Build history of the part. All positions in model axes, mm. A direction names the side the tool comes from. Round coordinates to 2 decimals unless told otherwise and drop trailing zeros. Loops run counter-clockwise (first coordinate to the right, second up) from the corner with the lowest first, then second, coordinate; pieces in that order, holes last. Notation, with made-up numbers: (-29, -5.5) - (-13, -5.5) arc R25 ccw to (-13, 27.5) - close; hole circle Ø8 at (-27, 45). An arc over 180 degrees is marked (long way). One line per question, with ' | ' between items. Start each with the question number.
Autodesk Inventor part; units mm, degrees
ref_plane "YZ Plane" through (0, 0, 0) normal (1, 0, 0) x (0, 1, 0)
ref_plane "XZ Plane" through (0, 0, 0) normal (0, 1, 0) x (-1, 0, 0)
ref_plane "XY Plane" through (0, 0, 0) normal (0, 0, 1) x (1, 0, 0)
sketch "Sketch1" plane through (0, 0, 0) normal (0, 0, 1) x (1, 0, 0)
  circle A0 centre (0, 0) radius 6
  dimension "d0" = 12
extrude "Extrusion1" add sketch "Sketch1" along normal blind 35
sketch "Sketch2" plane through (0, 0, 35) normal (0, 0, 1) x (1, 0, 0)
  circle A0 centre (0, 0) radius 2
  circle A1 centre (0, 0) radius 6
  dimension "d3" = 4
extrude "Extrusion2" cut sketch "Sketch2" against normal blind 5 contours A0
sketch "Sketch3" plane through (0, 0, 0) normal (0, 0, -1) x (-1, 0, 0)
  circle A0 centre (0, 0) radius 3.5
  dimension "d6" = 7
extrude "Extrusion3" cut sketch "Sketch3" against normal blind 2
properties part number "Laser" material "Aluminum 6061"
1) Tool access for faces 4 (the flat face through (3, 0, 35)), 5 (the flat face through (0, 0, 30)), 6 (the cylindrical face through (-3.233, -1.341, 0.986)): list every direction of +Z, -Z, +X, -X, +Y, -Y with a clear straight run to the whole face (end or side of a thin tool).
2) Saw through at A-A on y = 0. Write the cut outline in (x, z), and give its area (3 significant figures).
3) Saw through at D-D on z = 17. Write the cut outline in (x, y), and give its area (3 significant figures).
4) Two-plate mould, pull along Y, no slides. Class faces 1 (the flat face through (3, -3, 0)), 2 (the cylindrical face through (0, -2, 33)), 3 (the cylindrical face through (-6, 0, 17)): +Y half, -Y half, draft (parallel to the pull), parting line (faces both ways), or undercut.
5) Wall check: line 1 (Y direction, x = 0, z = 0.5); line 2 (Z direction, x = 2.5, y = -1.25); line 3 (Z direction, x = -1.75, y = -0.25). Give the ranges that are in metal, low to high. Write a range as [from, to].
6) Drop flat-ended pins along their axis: pin 1 (3 mm diameter, centred on x = -2, z = 25.5, fed in from -Y); pin 2 (2 mm diameter, centred on y = 3.5, z = 6.5, fed in from +X); pin 3 (3 mm diameter, centred on x = 0, y = 0, fed in from -Z). Give the stop position or say it passes through.
7) Saw through at C-C on z = 32.5. Write the cut outline in (x, y), and give its area (3 significant figures).
Answer key:
1) face 4: +Z, +X, -X, +Y, -Y | face 5: +Z | face 6: -Z
2) outline: (-6, 0) - (-3.5, 0) - (-3.5, 2) - (3.5, 2) - (3.5, 0) - (6, 0) - (6, 35) - (2, 35) - (2, 30) - (-2, 30) - (-2, 35) - (-6, 35) - close | area: 386 mm²
3) outline: circle Ø12 at (0, 0) | area: 113 mm²
4) face 1: draft | face 2: undercut | face 3: parting line
5) line 1: [-6, -3.5], [3.5, 6] | line 2: [2, 35] | line 3: [2, 30]
6) pin 1: y = -5.98 | pin 2: x = 5.45 | pin 3: z = 2
7) outline: circle Ø12 at (0, 0); hole circle Ø4 at (0, 0) | area: 101 mm²
